```python
from build123d import *

# Parameters (mm, degrees)
ESQUISSE1_W             = 102
ESQUISSE1_H             = 80
BOSS_EXTRU_1_DEPTH      = 1.5
ESQUISSE2_W             = 96
ESQUISSE2_H             = 76
BOSS_EXTRU_2_DEPTH      = 1.5
ESQUISSE3_R             = 1.75
ESQUISSE3_R_2           = 2
ESQUISSE3_R_3           = 3
ESQUISSE3_R_4           = 1.5
ENL_V_MAT_EXTRU_1_DEPTH = 5
BOSS_EXTRU_5_START      = 1
ESQUISSE6_W             = 21
ESQUISSE6_H             = 80
ESQUISSE6_R             = 1.75
BOSS_EXTRU_5_DEPTH      = 1
CHANFREIN2_SIZE         = 1
ESQUISSE7_W             = 21
ESQUISSE7_H             = 2.5
BOSS_EXTRU_6_DEPTH      = 1
ESQUISSE8_W             = 21
ESQUISSE8_H             = 2.5
BOSS_EXTRU_7_DEPTH      = 1


with BuildPart() as part:
    # Esquisse1 → Boss.-Extru.1 (new body)
    with BuildSketch(Plane(origin=(0, 0, 0), x_dir=(1, 0, 0), z_dir=(0, 1, 0))):
        with Locations((51, 40)):
            Rectangle(ESQUISSE1_W, ESQUISSE1_H)
    extrude(amount=BOSS_EXTRU_1_DEPTH)

    # Esquisse2 → Boss.-Extru.2 (add)
    with BuildSketch(Plane.XZ):
        with Locations((51, -40)):
            Rectangle(ESQUISSE2_W, ESQUISSE2_H)
    extrude(amount=BOSS_EXTRU_2_DEPTH)

    # Esquisse3 → Enl_v. mat.-Extru.1 (cut)
    with BuildSketch(Plane(origin=(0, 1.5, 0), x_dir=(1, 0, 0), z_dir=(0, 1, 0))):
        with Locations(Location((7, 74, 0), (0, 0, 270))):
            Circle(ESQUISSE3_R)
        with Locations(Location((7, 6, 0), (0, 0, 270))):
            Circle(ESQUISSE3_R)
        with Locations(Location((95, 6, 0), (0, 0, 270))):
            Circle(ESQUISSE3_R)
        with Locations(Location((95, 74, 0), (0, 0, 270))):
            Circle(ESQUISSE3_R)
        with Locations(Location((35, 72, 0), (0, 0, 270))):
            Circle(ESQUISSE3_R_2)
        with Locations(Location((50, 72, 0), (0, 0, 270))):
            Circle(ESQUISSE3_R_3)
        with Locations(Location((65, 72, 0), (0, 0, 270))):
            Circle(ESQUISSE3_R_4)
    extrude(amount=-ENL_V_MAT_EXTRU_1_DEPTH, mode=Mode.SUBTRACT)

    # Esquisse6 → Boss.-Extru.5 (add)
    # profile 1 of 2: a face of its own
    with BuildSketch(Plane(origin=(0, 1.5, 0), x_dir=(1, 0, 0), z_dir=(0, 1, 0)).offset(BOSS_EXTRU_5_START)):
        with Locations((91.5, 40)):
            Rectangle(ESQUISSE6_W, ESQUISSE6_H)
        with Locations(Location((95, 6, 0), (0, 0, 270))):
            Circle(ESQUISSE6_R, mode=Mode.SUBTRACT)
        with Locations(Location((95, 74, 0), (0, 0, 270))):
            Circle(ESQUISSE6_R, mode=Mode.SUBTRACT)
    # profile 2 of 2: a face of its own
    with BuildSketch(Plane(origin=(0, 1.5, 0), x_dir=(1, 0, 0), z_dir=(0, 1, 0)).offset(BOSS_EXTRU_5_START)):
        with Locations((10.5, 40)):
            Rectangle(ESQUISSE6_W, ESQUISSE6_H)
        with Locations(Location((7, 74, 0), (0, 0, 270))):
            Circle(ESQUISSE6_R, mode=Mode.SUBTRACT)
        with Locations(Location((7, 6, 0), (0, 0, 270))):
            Circle(ESQUISSE6_R, mode=Mode.SUBTRACT)
    extrude(amount=-BOSS_EXTRU_5_DEPTH)

    # Chanfrein2
    chanfrein2_edges = [part.edges().sort_by_distance(p)[0] for p in [
        (95, 2.5, -7.75),
        (95, 2.5, -75.75),
        (7, 2.5, -75.75),
        (7, 2.5, -7.75),
    ]]
    chamfer(chanfrein2_edges, length=CHANFREIN2_SIZE)

    # Esquisse7 → Boss.-Extru.6 (add)
    with BuildSketch(Plane.XY):
        with Locations((10.5, 1.25)):
            Rectangle(ESQUISSE7_W, ESQUISSE7_H)
        with Locations((91.5, 1.25)):
            Rectangle(ESQUISSE7_W, ESQUISSE7_H)
    extrude(amount=BOSS_EXTRU_6_DEPTH)

    # Esquisse8 → Boss.-Extru.7 (add)
    with BuildSketch(Plane(origin=(0, 0, -80), x_dir=(-1, 0, 0), z_dir=(0, 0, -1))):
        with Locations((-91.5, 1.25)):
            Rectangle(ESQUISSE8_W, ESQUISSE8_H)
        with Locations((-10.5, 1.25)):
            Rectangle(ESQUISSE8_W, ESQUISSE8_H)
    extrude(amount=BOSS_EXTRU_7_DEPTH)


solid = part.part
```
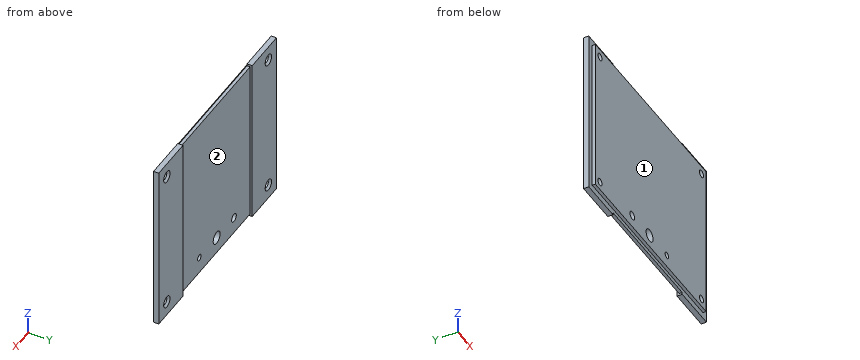
Check sheet for the modelled part. Datum: model origin and axes. Units: mm. Face numbers are marked on the shaded views. Round coordinates to 2 decimals unless told otherwise and drop trailing zeros. Loops run counter-clockwise (first coordinate to the right, second up) from the corner with the lowest first, then second, coordinate; pieces in that order, holes last. Notation, with made-up numbers: (72, -5) -> (116, -5) arc R21 cw to (116, 14) -> close; hole circle Ø2 at (11, 69.5). An arc over 180 degrees is marked (long way). Write item = value, one per line. Start each with the question number.
1) Gauge pin test, flat ends, axial feed: pin 1 Ø1.2 at (x, y) = (31, -0.5) entering from +Z; pin 2 Ø3 at (x, z) = (95, -74) entering from +Y; pin 3 Ø0.8 at (x, y) = (56.5, 1) entering from -Z; pin 4 Ø0.8 at (x, y) = (51.5, -1) entering from -Z. Record the tip position at first contact, or that the pin passes through.
2) Sectioned sample at C-C, the plane x = 50. Record the cut outline in (y, z), plus the area to 3 significant figures.
3) Thickness scan on probe 1 along X at (y, z) = (-0.3, -6); probe 2 along Z at (x, y) = (65, -0.3); probe 3 along Y at (x, z) = (79.5, -45). Record the ranges inside material, lowest first.
4) Sectioned sample at A-A, the plane x = 7. Record the cut outline in (y, z), plus the area to 3 significant figures.
5) Sectioned sample at D-D, the plane z = -6. Record the cut outline in (x, y), plus the area to 3 significant figures.
6) Release check for a two-part mould opening along X. For the marked faces 1 and 2 record: released by +X, released by -X, zero draft, split by the parting line, or undercut.
7) Sectioned sample at B-B, the plane y = -0.6. Record the cut outline in (x, z), plus the area to 3 significant figures.
Results are:
q1.pin_1 = 0
q1.pin_2 = through
q1.pin_3 = -80
q1.pin_4 = -78
q2.outline = (-1.5, -78) -> (0, -78) -> (0, -80) -> (1.5, -80) -> (1.5, -75) -> (-1.5, -75) -> close; (-1.5, -69) -> (1.5, -69) -> (1.5, 0) -> (0, 0) -> (0, -2) -> (-1.5, -2) -> close
q2.area = 216 mm^2
q3.probe_1 = 3 to 5.25, 8.75 to 93.25, 96.75 to 99
q3.probe_2 = -78 to -73.5, -70.5 to -2
q3.probe_3 = -1.5 to 1.5
q4.outline = (-1.5, -78) -> (0, -78) -> (0, -81) -> (2.5, -81) -> (2.5, -76.75) -> (1.5, -75.75) -> (-1.5, -75.75) -> close; (-1.5, -72.25) -> (1.5, -72.25) -> (2.5, -71.25) -> (2.5, -8.75) -> (1.5, -7.75) -> (-1.5, -7.75) -> close; (-1.5, -4.25) -> (1.5, -4.25) -> (2.5, -3.25) -> (2.5, 1) -> (0, 1) -> (0, -2) -> (-1.5, -2) -> close
q4.area = 289 mm^2
q5.outline = (0, 0) -> (3, 0) -> (3, -1.5) -> (5.25, -1.5) -> (5.25, 1.5) -> (4.25, 2.5) -> (0, 2.5) -> close; (8.75, -1.5) -> (93.25, -1.5) -> (93.25, 1.5) -> (92.25, 2.5) -> (81, 2.5) -> (81, 1.5) -> (21, 1.5) -> (21, 2.5) -> (9.75, 2.5) -> (8.75, 1.5) -> close; (96.75, -1.5) -> (99, -1.5) -> (99, 0) -> (102, 0) -> (102, 2.5) -> (97.75, 2.5) -> (96.75, 1.5) -> close
q5.area = 309 mm^2
q6.face_1 = zero draft
q6.face_2 = undercut
q7.outline = (3, -78) -> (99, -78) -> (99, -2) -> (3, -2) -> close; hole circle Ø3.5 at (7, -74); hole circle Ø3.5 at (7, -6); hole circle Ø4 at (35, -72); hole circle Ø6 at (50, -72); hole circle Ø3 at (65, -72); hole circle Ø3.5 at (95, -74); hole circle Ø3.5 at (95, -6)
q7.area = 7,210 mm^2
